The figure shows three views and two pictorial views of one solid part (mm, origin at its lowest corner). Answer the questions. Coordinates: 2 decimals unless noted, no trailing zeros. Loops run counter-clockwise (first coordinate to the right, second up) from the corner with the lowest first, then second, coordinate; pieces in that order, holes last.
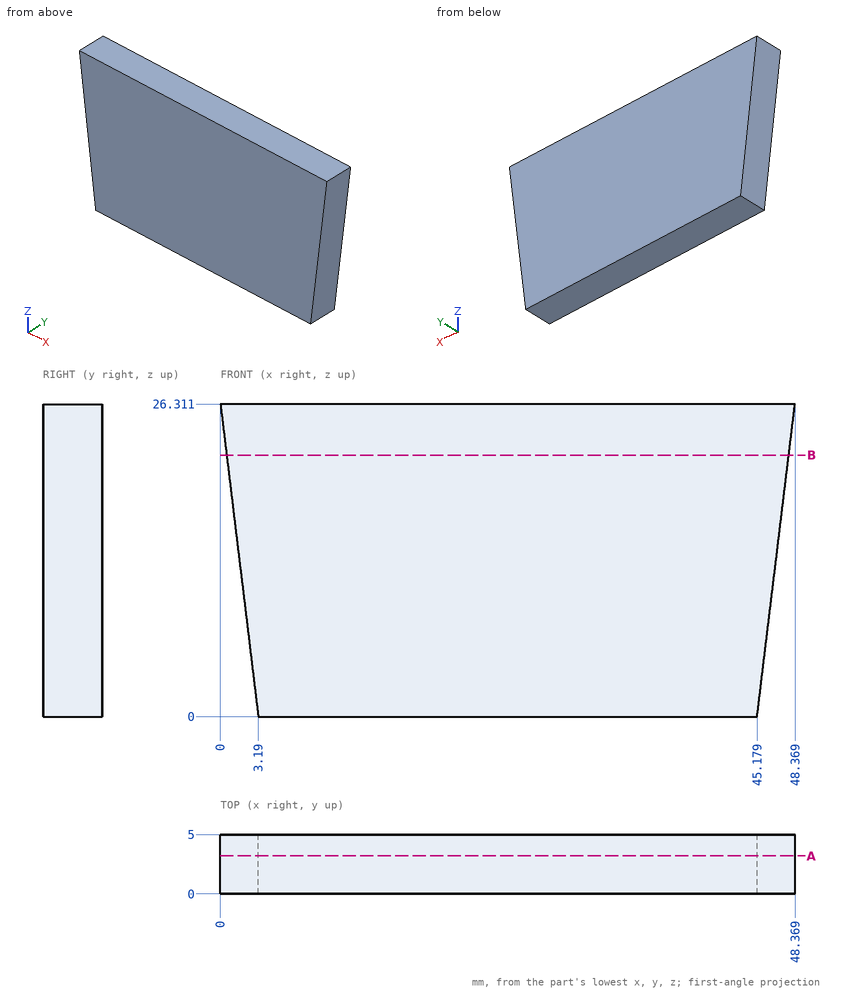
Q1. Flat-ended cylindrical pins translate along their axes: pin 1 Ø2 at (x, z) = (34, 7) entering from -Y; pin 2 Ø3 at (y, z) = (1, 11) entering from +X; pin 3 Ø1 at (y, z) = (2, 20.5) entering from -X; pin 4 Ø1.5 at (y, z) = (4, 14.5) entering from +X. Find the tip coordinate at first contact, or state that the pin passes through.
Findings below:
pin 1: stops at y = 0
pin 2: stops at x = 46.69
pin 3: stops at x = 0.64
pin 4: stops at x = 47.03
Q2. Straight lines are drawn through the part: probe 1 along X at (y, z) = (0.7, 12.75) (1 decimal); probe 2 along X at (y, z) = (3.1, 22.75). For each, find the intervals that lie inside material, in ascending order.
Findings below:
probe 1: x = 1.6 to 46.7
probe 2: x = 0.43 to 47.94
Q3. A cutting plane is placed at B-B (z = 22). Give the vertices of the cut face in (x, y), then the cut area to 3 significant figures.
Findings below:
outline: (0.52, 0) - (47.85, 0) - (47.85, 5) - (0.52, 5) - close
area: 237 mm2
Q4. A cutting plane is placed at A-A (y = 3.2). Give the vertices of the cut face in (x, z), then the cut area to 3 significant figures.
Findings below:
outline: (0, 26.31) - (3.19, 0) - (45.18, 0) - (48.37, 26.31) - close
area: 1,190 mm2
